Part model, mm, in its own coordinate system. Face numbers are marked on the shaded views. A direction names the side the tool comes from. Give positions to 0.01 mm unless a question says otherwise; leave off trailing zeros. Write each loop counter-clockwise with the first axis right and the second up, starting at its lowest first coordinate (ties: lowest second). Pieces come first, ordered by that corner, then holes. Notation, with made-up numbers: M 43,-6.5 L 102,-6.5 A17 cw 102,14.5 Z; hole C 42,47 d7. An arc over 180 degrees is marked long. Answer as CSV lines item,"result". Start each with the question number.
1) Mould opens along Z. For the marked faces 1, 2, 3 and 4 say: pulls with the +Z half, pulls with the -Z half, needs draft (parallel to the pull), parting line crosses it, or undercut.
2) Pin check, flat tips, straight feed: pin 1 Ø6 at (y, z) = (9.5, 4.5) entering from -X; pin 2 Ø6 at (x, y) = (2, 4.5) entering from -Z; pin 3 Ø3 at (x, y) = (8, 8) entering from +Z; pin 4 Ø3 at (x, z) = (6.5, 8) entering from +Y. Stop position of each tip, or through.
3) Wall check: line 1 along Z through (x, y) = (13, -7); line 2 along Z through (x, y) = (12.5, 10.5); line 3 along Y through (x, z) = (9, -1). Give the ranges that are in metal, low to high. Write a range as from..to.
4) Slice it at B-B, the plane y = 0. Give the cut face in (x, z), plus the area to 3 significant figures.
5) Slice it at C-C, the plane z = 12. Give the cut face in (x, y), plus the area to 3 significant figures.
6) Slice it at A-A, the plane z = 0. Give the cut face in (x, y), plus the area to 3 significant figures.
7) Tool access for the marked faces 5, 6, 7, 8 and 9: list every direction of +Z, -Z, +X, -X, +Y, -Y with a clear straight run to the whole face (end or side of a thin tool).
```python
from build123d import *

# Parameters (mm, degrees)
BASPROSKE_W        = 14
BASPROSKE_H        = 16
TOOTHCUT_DEPTH     = 27.608269391
TEETHCUTS_COUNT    = 14
TEETHCUTS_ANGLE    = 334.285714286
BORSKE_R           = 0.4
BORE_DEPTH         = 50.0000508
CUT_EXTRUDE1_DEPTH = 27.422624507


with BuildPart() as part:
    # BasProSke → Base-Revolve (revolve)
    with BuildSketch(Plane(origin=(0, 0, 0), x_dir=(1, 0, 0), z_dir=(0, 1, 0)), mode=Mode.PRIVATE) as base_revolve_sk:
        with Locations((7, 8)):
            Rectangle(BASPROSKE_W, BASPROSKE_H)
    revolve(base_revolve_sk.sketch.rotate(Axis((-10, 0, 0), (1, 0, 0)), 180), axis=Axis((-10, 0, 0), (1, 0, 0)))

    # TooCutSke → ToothCut (cut, through all)
    with BuildSketch(Plane(origin=(0, 0, 0), x_dir=(0, 0, -1), z_dir=(1, 0, 0))):
        with BuildLine():
            ThreePointArc((1.067858192, 11.449309144), (0, 11.499), (-1.067858192, 11.449309144))
            ThreePointArc((-1.067858192, 11.449309144), (-1.641684211, 13.812780716), (-3.163375005, 15.710076503))
            ThreePointArc((-3.163375005, 15.710076503), (0, 16.0254), (3.163375005, 15.710076503))
            ThreePointArc((3.163375005, 15.710076503), (1.641684211, 13.812780716), (1.067858192, 11.449309144))
        make_face()
    toothcut = extrude(amount=TOOTHCUT_DEPTH, mode=Mode.SUBTRACT)

    # TeethCuts: ToothCut ×14 about axis
    teethcuts_axis = Axis((-10, 0, 0), (1, 0, 0))
    for i in range(1, TEETHCUTS_COUNT):
        add(toothcut.rotate(teethcuts_axis, i * TEETHCUTS_ANGLE / (TEETHCUTS_COUNT - 1)), mode=Mode.SUBTRACT)

    # BorSke → Bore (cut, symmetric)
    with BuildSketch(Plane(origin=(0, 0, 0), x_dir=(0, 0, -1), z_dir=(1, 0, 0))):
        with Locations(Location((0, 0, 0), (0, 0, 180))):
            Circle(BORSKE_R)
    extrude(amount=BORE_DEPTH, both=True, mode=Mode.SUBTRACT)

    # Sketch1 → Cut-Extrude1 (cut, through all)
    with BuildSketch(Plane(origin=(14, 0, 0), x_dir=(0, 0, -1), z_dir=(1, 0, 0))):
        with BuildLine():
            Line((-5.291502622, 6), (5.291502622, 6))
            ThreePointArc((5.291502622, 6), (8, 0), (5.291502622, -6))
            Line((5.291502622, -6), (-5.291502622, -6))
            ThreePointArc((-5.291502622, -6), (-8, 0), (-5.291502622, 6))
        make_face()
    extrude(amount=-CUT_EXTRUDE1_DEPTH, mode=Mode.SUBTRACT)

    # Sketch3 → Cut-Revolve2 (revolve, cut)
    with BuildSketch(Plane(origin=(0, 0, 0), x_dir=(1, 0, 0), z_dir=(0, 1, 0)), mode=Mode.PRIVATE) as cut_revolve2_sk:
        Polygon((0, 0), (2.289763839, 0), (2.289763839, 9), (-2.541437219, 11.109912375), (-2.541437219, 0), align=None)
    revolve(cut_revolve2_sk.sketch.rotate(Axis((-21.436119779, 0, 0), (1, 0, 0)), 180), axis=Axis((-21.436119779, 0, 0), (1, 0, 0)), mode=Mode.SUBTRACT)


solid = part.part
```
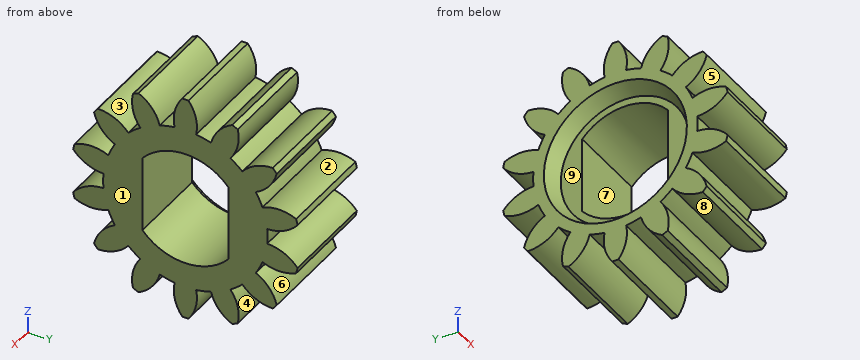
Found:
1,face 1,"needs draft"
1,face 2,"undercut"
1,face 3,"pulls with the +Z half"
1,face 4,"undercut"
2,pin 1,"x = 0"
2,pin 2,"z = -14.6"
2,pin 3,"z = 14.6"
2,pin 4,"y = 12.74"
3,line 1,"-14.39..-10.8, -9.12..9.12, 10.8..14.39"
3,line 2,"-10.02..-6.31, -4.69..4.69, 6.31..10.02"
3,line 3,"-11.46..-6, 6..11.46"
4,outline,"M 0,-16 L 14,-16 L 14,-8 L 2.29,-8 L 2.29,-9 L 0,-10 Z; M 0,10 L 2.29,9 L 2.29,8 L 14,8 L 14,16 L 0,16 Z"
4,area,"217 mm²"
5,outline,"M 0,-7.36 L 14,-7.36 L 14,-3.98 L 0,-3.98 Z; M 0,-1.6 L 14,-1.6 L 14,1.6 L 0,1.6 Z; M 0,3.98 L 14,3.98 L 14,7.36 L 0,7.36 Z"
5,area,"140 mm²"
6,outline,"M 0,-11.5 L 14,-11.5 L 14,-6 L 2.29,-6 L 2.29,-9 L 0,-10 Z; M 0,10 L 2.29,9 L 2.29,6 L 14,6 L 14,11.5 L 0,11.5 Z"
6,area,"138 mm²"
7,face 5,"+X, -X, -Y"
7,face 6,"+X, -X, +Y"
7,face 7,"+X, -X"
7,face 8,"-Z, +X, -X"
7,face 9,"-X"
